```python
from build123d import *

# Parameters (mm, degrees)
BOSS_EXTRUDE1_DEPTH      = 415.2
BOSS_EXTRUDE1_DEPTH_BACK = 415.2
CUT_EXTRUDE1_DEPTH       = 33
CUT_EXTRUDE2_DEPTH       = 33


with BuildPart() as part:
    # Sketch1 → Boss-Extrude1 (new body, two sides)
    with BuildSketch(Plane.XY) as boss_extrude1_sk:
        with BuildLine():
            Line((-14, -16), (14, -16))
            ThreePointArc((14, -16), (15.414213562, -15.414213562), (16, -14))
            Line((16, -14), (16, 14))
            ThreePointArc((16, 14), (15.414213562, 15.414213562), (14, 16))
            Line((14, 16), (-14, 16))
            ThreePointArc((-14, 16), (-15.414213562, 15.414213562), (-16, 14))
            Line((-16, 14), (-16, -14))
            ThreePointArc((-16, -14), (-15.414213562, -15.414213562), (-14, -16))
        make_face()
        with BuildLine():
            Line((-14, 14.48), (14, 14.48))
            ThreePointArc((14, 14.48), (14.339411255, 14.339411255), (14.48, 14))
            Line((14.48, 14), (14.48, -14))
            ThreePointArc((14.48, -14), (14.339411255, -14.339411255), (14, -14.48))
            Line((14, -14.48), (-14, -14.48))
            ThreePointArc((-14, -14.48), (-14.339411255, -14.339411255), (-14.48, -14))
            Line((-14.48, -14), (-14.48, 14))
            ThreePointArc((-14.48, 14), (-14.339411255, 14.339411255), (-14, 14.48))
        make_face(mode=Mode.SUBTRACT)
    extrude(amount=BOSS_EXTRUDE1_DEPTH)
    extrude(boss_extrude1_sk.sketch, amount=-BOSS_EXTRUDE1_DEPTH_BACK)

    # Sketch2 → Cut-Extrude1 (cut, through all)
    with BuildSketch(Plane(origin=(16, 0, 0), x_dir=(0, 0, -1), z_dir=(1, 0, 0))):
        Polygon((-415.2, -16), (-415.2, 16), (-363.609390927, 16), align=None)
    extrude(amount=-CUT_EXTRUDE1_DEPTH, mode=Mode.SUBTRACT)

    # Sketch3 → Cut-Extrude2 (cut, through all)
    with BuildSketch(Plane(origin=(16, 0, 0), x_dir=(0, 0, -1), z_dir=(1, 0, 0))):
        Polygon((415.2, 16), (415.2, -16), (395.351426424, 16), align=None)
    extrude(amount=-CUT_EXTRUDE2_DEPTH, mode=Mode.SUBTRACT)


solid = part.part
```
Work out the finished part from the listing and answer in its coordinate system (mm). A direction names the side the tool comes from. Give positions to 0.01 mm unless a question says otherwise; leave off trailing zeros. Order: outer loops, then holes, each group sorted by start corner. A loop starts at its lowest first (then second) coordinate and runs counter-clockwise, first axis right, second up. Notation, with made-up numbers: M -30.75,-3.5 L -17.75,-3.5 A27 ccw -17.75,18.5 Z; hole C 14.25,71.25 d2. An arc over 180 degrees is marked long. Return JSON: item names as keys, results as strings.
1) Straight lines are drawn through the part: line 1 along Y through (x, z) = (12.5, -238); line 2 along Y through (x, z) = (15, -93). For each, find the intervals that lie inside material, in ascending order. Write a range as [from, to].
Resolved:
{"line 1": "[-16, -14.48], [14.48, 16]", "line 2": "[-15.73, 15.73]"}
2) Section A-A, the plane z = -307 is taken. Write down the section's boundary in (x, y).
Resolved:
{"outline": "M -16,-14 A2 ccw -14,-16 L 14,-16 A2 ccw 16,-14 L 16,14 A2 ccw 14,16 L -14,16 A2 ccw -16,14 Z; hole M -14.48,-14 A0.48 ccw -14,-14.48 L 14,-14.48 A0.48 ccw 14.48,-14 L 14.48,14 A0.48 ccw 14,14.48 L -14,14.48 A0.48 ccw -14.48,14 Z"}
3) This flat-tipped pin is pushed along its axis until it touches: pin 1 (2 mm diameter, centred on x = 11.5, y = -2, fed in from +Z). Where does it stop, or does it pass through?
Resolved:
{"pin 1": "through"}
4) Section C-C, the plane y = 4 is taken. Write down the section's boundary in (x, z), plus the area to 3 significant figures.
Resolved:
{"outline": "M -16,-402.79 L -14.48,-402.79 L -14.48,382.96 L -16,382.96 Z; M 14.48,-402.79 L 16,-402.79 L 16,382.96 L 14.48,382.96 Z", "area": "2,390 mm^2"}
5) A tool of negligible diameter and unlimited length cuts with its end or side. For faces 5 (the flat face through (-15.33, -0.07, -405.32)), 6 (the flat face through (14.48, 0, 5)), from which of +Z, -Z, +X, -X, +Y, -Y can it reach the whole face along a straight path? Write none if from no direction.
Resolved:
{"face 5": "-Z, +X, -X, +Y", "face 6": "+Z, -Z"}
6) Section B-B, the plane x = 2.5 is taken. Write down the section's boundary in (y, z).
Resolved:
{"outline": "M -16,-415.2 L -14.48,-414.26 L -14.48,412.75 L -16,415.2 Z; M 14.48,-396.29 L 16,-395.35 L 16,363.61 L 14.48,366.06 Z"}
7) For a pull along Y with two mould halves and no side action, classify faces 1 (the flat face through (-15.333, 0.075, 389.284)), 2 (the flat face through (0, -16, 6)), 3 (the flat face through (-16, 0, 5)), 4 (the flat face through (-14.48, 0, 5)) as +Y half, -Y half, draft (parallel to the pull), parting line (faces both ways), or undercut.
Resolved:
{"face 1": "+Y half", "face 2": "-Y half", "face 3": "draft", "face 4": "undercut"}
